from build123d import *

# Parameters (mm, degrees)
F0_R     = 176.2125
F0_R_2   = 4.7625
F1_DEPTH = 7.9375


with BuildPart() as f1:
    # F0 (on Front) → F1 (new body)
    with BuildSketch(Plane.XZ):
        Circle(F0_R)
        with Locations((0, -144.4625)):
            Circle(F0_R_2, mode=Mode.SUBTRACT)
        with Locations((-144.4625, 0)):
            Circle(F0_R_2, mode=Mode.SUBTRACT)
        Circle(F0_R_2, mode=Mode.SUBTRACT)
        with Locations((144.4625, 0)):
            Circle(F0_R_2, mode=Mode.SUBTRACT)
        with Locations((0, 144.4625)):
            Circle(F0_R_2, mode=Mode.SUBTRACT)
    extrude(amount=F1_DEPTH)


solid = f1.part
Verification items for the finished model (mm, model axes). Give positions to 0.01 mm unless a question says otherwise; leave off trailing zeros. Loops run counter-clockwise (first coordinate to the right, second up) from the corner with the lowest first, then second, coordinate; pieces in that order, holes last. Notation, with made-up numbers: (2.25, -6) - (37.25, -6) arc R32 cw to (37.25, 24) - close; hole circle Ø8 at (-23, 51). An arc over 180 degrees is marked (long way). Write item = value, one per line. Start each with the question number.
Q1. Cross-section at C-C, the plane y = -3.25. Enter the section's corners in (x, z) (1 decimal), and give its area (3 significant figures).
Q2. Cross-section at A-A, the plane z = 0. Enter the section's corners in (x, y) (1 decimal), and give its area (3 significant figures).
Q3. Depth check by flat-ended pin: P1, Ø1.5, axis at y = -6.5, z = 68.5, coming from the -X side; P2, Ø4, axis at y = -4, z = 12.5, coming from the -X side; P3, Ø3, axis at x = -136.5, y = -4, coming from the +Z side. Enter the tip coordinate at first touch or a pass-through.
Q4. Mould release check, pull along X, two halves, no side actions. Record for faces 1 (the face through (37, -7.938, 2)), 2 (the face through (-1.032, -3.913, -149.112)), 3 (the face through (-3.78, -3.91, -2.9)), 4 (the face through (94.731, -3.913, 148.583)): released by +X, released by -X, zero draft, split by the parting line, or undercut.
Q5. Cross-section at B-B, the plane x = 0. Enter the section's corners in (y, z) (1 decimal), and give its area (3 significant figures).
Q6. Thickness scan on line 1 (Z direction, x = 0, y = -5) (1 decimal); line 2 (Z direction, x = 144, y = -5.75); line 3 (X direction, y = -3.75, z = 143). Record the ranges inside material, lowest first.
Q7. Cross-section at D-D, the plane z = 98.5. Enter the section's corners in (x, y), and give its area (3 significant figures).
Answer key:
q1.outline = circle Ø352.4 at (0, 0); hole circle Ø9.5 at (-144.5, 0); hole circle Ø9.5 at (0, -144.5); hole circle Ø9.5 at (0, 0); hole circle Ø9.5 at (0, 144.5); hole circle Ø9.5 at (144.5, 0)
q1.area = 97,200 mm^2
q2.outline = (-176.2, -7.9) - (-149.2, -7.9) - (-149.2, 0) - (-176.2, 0) - close; (-139.7, -7.9) - (-4.8, -7.9) - (-4.8, 0) - (-139.7, 0) - close; (4.8, -7.9) - (139.7, -7.9) - (139.7, 0) - (4.8, 0) - close; (149.2, -7.9) - (176.2, -7.9) - (176.2, 0) - (149.2, 0) - close
q2.area = 2,570 mm^2
q3.P1 = -162.67
q3.P2 = -175.9
q3.P3 = 113.25
q4.face_1 = zero draft
q4.face_2 = undercut
q4.face_3 = undercut
q4.face_4 = split by the parting line
q5.outline = (-7.9, -176.2) - (0, -176.2) - (0, -149.2) - (-7.9, -149.2) - close; (-7.9, -139.7) - (0, -139.7) - (0, -4.8) - (-7.9, -4.8) - close; (-7.9, 4.8) - (0, 4.8) - (0, 139.7) - (-7.9, 139.7) - close; (-7.9, 149.2) - (0, 149.2) - (0, 176.2) - (-7.9, 176.2) - close
q5.area = 2,570 mm^2
q6.line_1 = -176.2 to -149.2, -139.7 to -4.8, 4.8 to 139.7, 149.2 to 176.2
q6.line_2 = -101.56 to -4.74, 4.74 to 101.56
q6.line_3 = -102.97 to -4.53, 4.53 to 102.97
q7.outline = (-146.11, -7.94) - (146.11, -7.94) - (146.11, 0) - (-146.11, 0) - close
q7.area = 2,320 mm^2
